Part model, mm, in its own coordinate system. A direction names the side the tool comes from. Coordinates: 2 decimals unless noted, no trailing zeros. Loops run counter-clockwise (first coordinate to the right, second up) from the corner with the lowest first, then second, coordinate; pieces in that order, holes last. Notation, with made-up numbers: (7, 55) -> (49, 55) arc R22 ccw to (49, 90) -> close; hole circle Ø9 at (77, 61.5). An arc over 180 degrees is marked (long way). One line per question, with ' | ' between items. Start each with the question number.
1) Cut at B-B (z = -6.25). List the corners of the cut face in (x, y).
2) Cut at C-C (z = 0.25). List the corners of the cut face in (x, y).
3) Probe L1, parallel to Z at x = -0.1, y = -0.3; L2, parallel to Z at x = 0.95, y = -1.65; L3, parallel to Y at x = 0.55, z = -4. List the from-to ranges inside material, lowest first. Write a range as from..to.
4) Two-plate mould, pull along Y, no slides. Class faces 4 (the face through (-0.596, 2.685, 1.486)), 5 (the face through (0, 0, -10)), 6 (the face through (1.25, 0, 2)): released by +Y, released by -Y, zero draft, split by the parting line, or undercut.
5) Cut at A-A (y = 0). List the corners of the cut face in (x, z), plus the area to 3 significant figures.
6) Drop flat-ended pins along their axis: pin 1 (3 mm diameter, centred on y = 1, z = -3.5, fed in from +X); pin 2 (0.6 mm diameter, centred on x = 0, y = 0.5, fed in from +Z); pin 3 (3 mm diameter, centred on y = 1.5, z = -3, fed in from -X). Give the stop position or say it passes through.
7) 3-axis set-ups, long thin cutter, end or side, ignore diameter. For faces 1 (the face through (0, 2, 3)), 2 (the face through (-2, 0, 0)), 3 (the face through (-0.618, -1.086, 2.256)): which of +Z, -Z, +X, -X, +Y, -Y reach the whole face in a straight line?
Autodesk Inventor part; units mm, degrees
ref_plane "YZ Plane" through (0, 0, 0) normal (1, 0, 0) x (0, 1, 0)
ref_plane "XZ Plane" through (0, 0, 0) normal (0, 1, 0) x (-1, 0, 0)
ref_plane "XY Plane" through (0, 0, 0) normal (0, 0, 1) x (1, 0, 0)
sketch "スケッチ1" plane through (0, 0, 0) normal (0, 0, 1) x (1, 0, 0)
  circle A0 centre (0, 0) radius 2.75
  dimension "d0" = 5.5
extrude "押し出し1" add sketch "スケッチ1" along normal blind 3
sketch "スケッチ2" plane through (0, 0, 0) normal (0, 0, -1) x (-1, 0, 0)
  circle A0 centre (0, 0) radius 2.75
  circle A1 centre (0, 0) radius 1.5
  dimension "d3" = 3
extrude "押し出し2" add sketch "スケッチ2" along normal blind 10 contours A1
sketch "スケッチ3" plane through (0, 0, 3) normal (0, 0, 1) x (1, 0, 0)
  circle A0 centre (0, 0) radius 2.75
  line L0 (0, 1.4434) -> (1.25, 0.7217)
  line L1 (1.25, 0.7217) -> (1.25, -0.7217)
  line L2 (1.25, -0.7217) -> (0, -1.4434)
  line L3 (0, -1.4434) -> (-1.25, -0.7217)
  line L4 (-1.25, -0.7217) -> (-1.25, 0.7217)
  line L5 (-1.25, 0.7217) -> (0, 1.4434)
  dimension "d6" = 1.25
extrude "押し出し3" cut sketch "スケッチ3" against normal blind 1.5 contours L0 L1 L2 L3 L4 L5
fillet "フィレット1" radius 0.5 2 edges at (-2.75, 0, 3) (-2.75, 0, 0)
fillet "フィレット2" radius 0.3 19 edges at (-0.625, 1.0825, 3) (-1.25, 0, 3) (-0.625, -1.0825, 3) (0.625, -1.0825, 3) (1.25, 0, 3) (0.625, 1.0825, 3) (-0.625, 1.0825, 1.5) (0.625, 1.0825, 1.5) (0, 1.4434, 2.25) (-1.25, 0.7217, 2.25) (-0.625, -1.0825, 1.5) (-1.25, -0.7217, 2.25) (-1.25, 0, 1.5) (1.25, 0, 1.5) (1.25, 0.7217, 2.25) (1.25, -0.7217, 2.25) (0.625, -1.0825, 1.5) (0, -1.4434, 2.25) (1.5, 0, -10)
thread "ねじ2"
Reported:
1) outline: circle Ø3 at (0, 0)
2) outline: circle Ø5.37 at (0, 0)
3) L1: z = -10..1.5 | L2: z = 0..3 | L3: y = -1.4..1.4
4) face 4: split by the parting line | face 5: zero draft | face 6: undercut
5) outline: (-2.75, 0.5) arc R0.5 ccw to (-2.25, 0) -> (-1.5, 0) -> (-1.5, -9.7) arc R0.3 ccw to (-1.2, -10) -> (1.2, -10) arc R0.3 ccw to (1.5, -9.7) -> (1.5, 0) -> (2.25, 0) arc R0.5 ccw to (2.75, 0.5) -> (2.75, 2.5) arc R0.5 ccw to (2.25, 3) -> (1.55, 3) arc R0.3 ccw to (1.25, 2.7) -> (1.25, 1.8) arc R0.3 cw to (0.95, 1.5) -> (-0.95, 1.5) arc R0.3 cw to (-1.25, 1.8) -> (-1.25, 2.7) arc R0.3 ccw to (-1.55, 3) -> (-2.25, 3) arc R0.5 ccw to (-2.75, 2.5) -> close | area: 42.5 mm²
6) pin 1: stops at x = 1.5 | pin 2: stops at z = 1.5 | pin 3: stops at x = -1.5
7) face 1: +Z, +X, -X, +Y, -Y | face 2: -Z | face 3: +Z
